Geometry check sheet. Reference: drawing and pictorial views, mm from the part's lowest x, y, z. Coordinates: 2 decimals unless noted, no trailing zeros. Order: outer loops, then holes, each group sorted by start corner. A loop starts at its lowest first (then second) coordinate and runs counter-clockwise, first axis right, second up. Notation, with made-up numbers: M -2.5,80.5 L 45.5,80.5 A16 ccw 45.5,104.5 Z; hole C 27,77 d3. An arc over 180 degrees is marked long. Return JSON: item names as keys, results as strings.
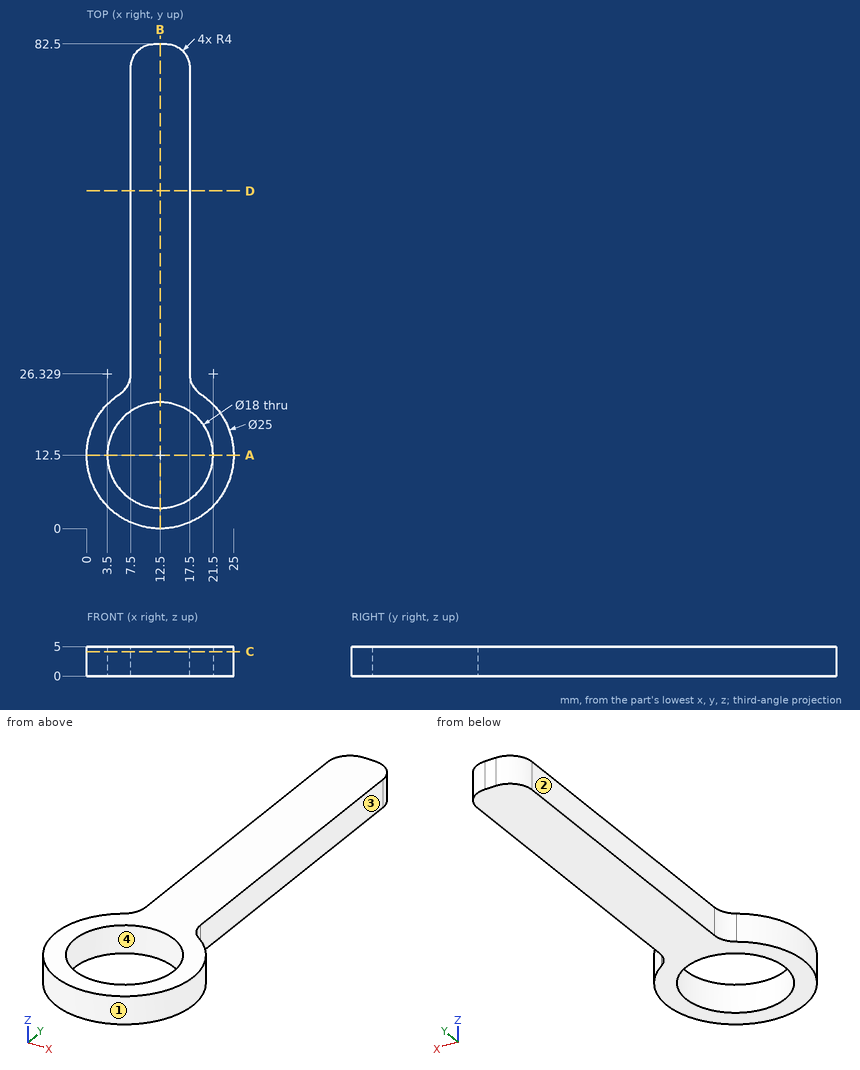
Q1. Cross-section at B-B, the plane x = 12.5. Record the boundary of the cut face in (y, z).
Values:
{"outline": "M 0,0 L 3.5,0 L 3.5,5 L 0,5 Z; M 21.5,0 L 82.5,0 L 82.5,5 L 21.5,5 Z"}
Q2. Material ranges on line 1 along Y through (x, z) = (12.5, 1.15); line 2 along X through (y, z) = (46, 3.35); line 3 along Y through (x, z) = (18.5, 0.5) (1 decimal), recorded low to high.
Values:
{"line 1": "0 to 3.5, 21.5 to 82.5", "line 2": "7.5 to 17.5", "line 3": "1.5 to 5.8, 19.2 to 23.7"}
Q3. Go/stop test with flat-tipped pins: pin 1 (1 mm diameter, centred on x = 16.5, z = 4, fed in from -Y); pin 2 (1.5 mm diameter, centred on x = 4.5, z = 3, fed in from +Y); pin 3 (1 mm diameter, centred on y = 39, z = 3.5, fed in from +X); pin 4 (3 mm diameter, centred on x = 12, y = 45.5, fed in from -Z). Record where each tip stops, or that it passes through.
Values:
{"pin 1": "y = 0.5", "pin 2": "y = 22.68", "pin 3": "x = 17.5", "pin 4": "z = 0"}
Q4. Cross-section at C-C, the plane z = 4.15. Record the boundary of the cut face in (x, y).
Values:
{"outline": "M 5.68,22.98 A12.5 ccw long 19.32,22.98 A4 cw 17.5,26.33 L 17.5,78.5 A4 ccw 13.5,82.5 L 11.5,82.5 A4 ccw 7.5,78.5 L 7.5,26.33 A4 cw Z; hole C 12.5,12.5 d18"}
Q5. Draft check along X on the marked faces 1, 2, 3 and 4. Enter one of: pulls with the +X half, pulls with the -X half, needs draft (parallel to the pull), parting line crosses it, or undercut.
Values:
{"face 1": "parting line crosses it", "face 2": "pulls with the -X half", "face 3": "pulls with the +X half", "face 4": "undercut"}
Q6. Cross-section at D-D, the plane y = 57.5. Record the boundary of the cut face in (x, z).
Values:
{"outline": "M 7.5,0 L 17.5,0 L 17.5,5 L 7.5,5 Z"}
Q7. Cross-section at A-A, the plane y = 12.5. Record the boundary of the cut face in (x, z).
Values:
{"outline": "M 0,0 L 3.5,0 L 3.5,5 L 0,5 Z; M 21.5,0 L 25,0 L 25,5 L 21.5,5 Z"}
